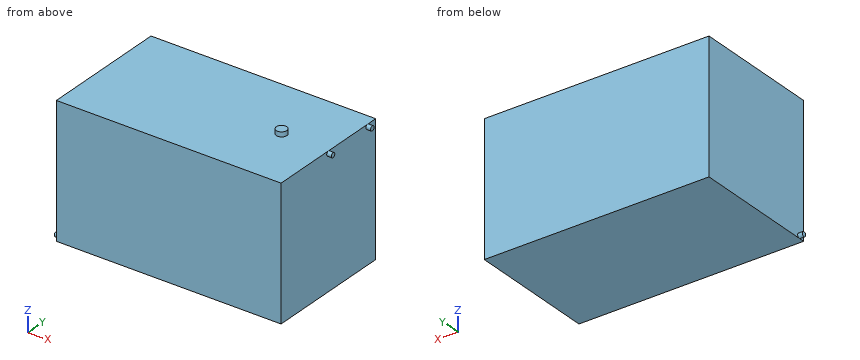
from build123d import *

# Parameters (mm, degrees)
F0_W     = 609.6
F0_H     = 349.25
F1_DEPTH = 355.6
F3_DEPTH = 12.7
F4_R     = 6.35
F5_DEPTH = 12.7
F6_R     = 6.35
F7_DEPTH = 12.7


with BuildPart() as f1:
    # F0 (on Top) → F1 (new body)
    with BuildSketch(Plane.XY):
        with Locations((-304.8, 174.625)):
            Rectangle(F0_W, F0_H)
    extrude(amount=F1_DEPTH)

    # F2 (on face) → F3 (join)
    with BuildSketch(Plane.XY.offset(355.6)):
        with BuildLine():
            ThreePointArc((-141.2875, 174.625), (-127, 160.3375), (-112.7125, 174.625))
            ThreePointArc((-112.7125, 174.625), (-127, 188.9125), (-141.2875, 174.625))
        make_face()
    extrude(amount=F3_DEPTH)

    # F4 (on face) → F5 (join)
    with BuildSketch(Plane.YZ):
        with Locations((174.625, 349.25)):
            Circle(F4_R)
        with Locations((319.281042, 349.25)):
            Circle(F4_R)
    extrude(amount=F5_DEPTH)

    # F6 (on face) → F7 (join)
    with BuildSketch(Plane(origin=(-609.6, 0, 0), x_dir=(0, -1, 0), z_dir=(-1, 0, 0))):
        with Locations((-15.958672, 6.35)):
            Circle(F6_R)
    extrude(amount=F7_DEPTH)


solid = f1.part
Can you work these out from the model? Positions are in its coordinate system, mm. Give positions to 0.01 mm unless a question says otherwise; leave off trailing zeros. Order: outer loops, then holes, each group sorted by start corner. A loop starts at its lowest first (then second) coordinate and runs counter-clockwise, first axis right, second up. Notation, with made-up numbers: M 36,31 L 91,31 A5 cw 91,36 Z; hole C 5.5,22.5 d10. An arc over 180 degrees is marked long. Use a Markdown table: item, result. Add a question column.
Item 1: Suppose I cut it at B-B (y = 212). List the corners of the cut face in (x, z) for me.
Item 2: Will these pins go through, and if not, where does the flat tip stop? pin 1 (10 mm diameter, centred on y = 295, z = 105, fed in from +X); pin 2 (1.5 mm diameter, centred on x = -390, y = 160, fed in from +Z); pin 3 (3 mm diameter, centred on y = 166.5, z = 173, fed in from -X).
Item 3: Suppose I cut it at A-A (x = -127). List the corners of the cut face in (y, z) for me.
Item 4: If I drill on L1, parallel to Z at x = -530.5, y = 330.5; L2, parallel to X at y = 26, z = 20, over which ranges is the centre line in solid material (lowest first)? Write a range as [from, to].
Item 5: Suppose I cut it at C-C (z = 224). List the corners of the cut face in (x, y) for me, then the cut area to 3 significant figures.
Answer sheet:
| question | item | result |
|---|---|---|
| 1 | outline | M -609.6,0 L 0,0 L 0,355.6 L -609.6,355.6 Z |
| 2 | pin 1 | stops at x = 0 |
| 2 | pin 2 | stops at z = 355.6 |
| 2 | pin 3 | stops at x = -609.6 |
| 3 | outline | M 0,0 L 349.25,0 L 349.25,355.6 L 188.91,355.6 L 188.91,368.3 L 160.34,368.3 L 160.34,355.6 L 0,355.6 Z |
| 4 | L1 | z = [0, 355.6] |
| 4 | L2 | x = [-609.6, 0] |
| 5 | outline | M -609.6,0 L 0,0 L 0,349.25 L -609.6,349.25 Z |
| 5 | area | 213,000 mm² |
